```python
from build123d import *

# Parameters (mm, degrees)
SKETCH2_W                = 177.8
SKETCH2_H                = 165.1
BOSS_EXTRUDE1_DEPTH      = 25.4
SKETCH6_W                = 25.4
SKETCH6_H                = 25.4
BOSS_EXTRUDE2_DEPTH      = 31.75
MIRROR2_COPY_1_SKETCH_W  = 25.4
MIRROR2_COPY_1_SKETCH_H  = 25.4
MIRROR2_COPY_1_DEPTH     = 31.75
SKETCH9_W                = 107.188
SKETCH9_H                = 107.188
CUT_EXTRUDE3_DEPTH       = 3.556
SKETCH10_RX              = 2.159
SKETCH10_RY              = 2.159
CUT_EXTRUDE4_DEPTH       = 20.32
MIRROR4_COPY_1_SKETCH_RX = 2.159
MIRROR4_COPY_1_SKETCH_RY = 2.159
MIRROR4_COPY_1_DEPTH     = 20.32
SKETCH14_R               = 5.08
CUT_EXTRUDE5_DEPTH       = 20.32
MIRROR6_COPY_1_SKETCH_R  = 5.08
MIRROR6_COPY_1_DEPTH     = 20.32


with BuildPart() as part:
    # Sketch2 → Boss-Extrude1 (new body)
    with BuildSketch(Plane(origin=(0, 0, 0), x_dir=(1, 0, 0), z_dir=(0, 1, 0))):
        with Locations((88.9, -82.55)):
            Rectangle(SKETCH2_W, SKETCH2_H)
    extrude(amount=BOSS_EXTRUDE1_DEPTH)

    # Sketch6 → Boss-Extrude2 (add)
    with BuildSketch(Plane(origin=(0, 25.4, 0), x_dir=(1, 0, 0), z_dir=(0, 1, 0))):
        with Locations((12.7, -12.7)):
            Rectangle(SKETCH6_W, SKETCH6_H)
    boss_extrude2 = extrude(amount=BOSS_EXTRUDE2_DEPTH)

    # Mirror1: Boss-Extrude2 across plane
    add(boss_extrude2.mirror(Plane(origin=(0, 0, 82.55), x_dir=(1, 0, 0), z_dir=(0, 0, -1))))

    # Mirror2: Boss-Extrude2 across plane
    add(boss_extrude2.mirror(Plane.ZY.offset(-88.9)))

    # Mirror2 copy 1 sketch → Mirror2 copy 1 (add)
    with BuildSketch(Plane(origin=(177.8, 25.4, 165.1), x_dir=(-1, 0, 0), z_dir=(0, 1, 0))):
        with Locations((12.7, -12.7)):
            Rectangle(MIRROR2_COPY_1_SKETCH_W, MIRROR2_COPY_1_SKETCH_H)
    extrude(amount=MIRROR2_COPY_1_DEPTH)

    # Sketch9 → Cut-Extrude3 (cut)
    with BuildSketch(Plane(origin=(0, 25.4, 0), x_dir=(1, 0, 0), z_dir=(0, 1, 0))):
        with Locations((59.944, -81.276983136)):
            Rectangle(SKETCH9_W, SKETCH9_H)
    extrude(amount=-CUT_EXTRUDE3_DEPTH, mode=Mode.SUBTRACT)

    # Sketch10 → Cut-Extrude4 (cut)
    with BuildSketch(Plane(origin=(0, 21.844, 0), x_dir=(1, 0, 0), z_dir=(0, 1, 0))):
        with Locations(Location((9.662951288, -31.573935809), (0, 0, 56.28607255))):
            Ellipse(SKETCH10_RX, SKETCH10_RY)
    cut_extrude4 = extrude(amount=-CUT_EXTRUDE4_DEPTH, mode=Mode.SUBTRACT)

    # Mirror3: Cut-Extrude4 across plane
    add(cut_extrude4.mirror(Plane.XY.offset(81.276983136)), mode=Mode.SUBTRACT)

    # Mirror4: Cut-Extrude4 across plane
    add(cut_extrude4.mirror(Plane.ZY.offset(-59.944)), mode=Mode.SUBTRACT)

    # Mirror4 copy 1 sketch → Mirror4 copy 1 (cut)
    with BuildSketch(Plane(origin=(119.888, 21.844, 162.553966273), x_dir=(-1, 0, 0), z_dir=(0, 1, 0))):
        with Locations(Location((9.662951288, -31.573935809), (0, 0, 56.28607255))):
            Ellipse(MIRROR4_COPY_1_SKETCH_RX, MIRROR4_COPY_1_SKETCH_RY)
    extrude(amount=-MIRROR4_COPY_1_DEPTH, mode=Mode.SUBTRACT)

    # Sketch14 → Cut-Extrude5 (cut)
    with BuildSketch(Plane(origin=(0, 57.15, 0), x_dir=(1, 0, 0), z_dir=(0, 1, 0))):
        with Locations(Location((12.7, -12.7, 0), (0, 0, 270))):
            Circle(SKETCH14_R)
    cut_extrude5 = extrude(amount=-CUT_EXTRUDE5_DEPTH, mode=Mode.SUBTRACT)

    # Mirror5: Cut-Extrude5 across plane
    add(cut_extrude5.mirror(Plane.ZY.offset(-88.9)), mode=Mode.SUBTRACT)

    # Mirror6: Cut-Extrude5 across plane
    add(cut_extrude5.mirror(Plane(origin=(0, 0, 82.55), x_dir=(1, 0, 0), z_dir=(0, 0, -1))), mode=Mode.SUBTRACT)

    # Mirror6 copy 1 sketch → Mirror6 copy 1 (cut)
    with BuildSketch(Plane(origin=(177.8, 57.15, 165.1), x_dir=(-1, 0, 0), z_dir=(0, 1, 0))):
        with Locations(Location((12.7, -12.7, 0), (0, 0, 270))):
            Circle(MIRROR6_COPY_1_SKETCH_R)
    extrude(amount=-MIRROR6_COPY_1_DEPTH, mode=Mode.SUBTRACT)


solid = part.part
```
Could you check a few things on this model? Use its own coordinates, in mm. A direction names the side the tool comes from. Give positions to 0.01 mm unless a question says otherwise; leave off trailing zeros. Write each loop counter-clockwise with the first axis right and the second up, starting at its lowest first coordinate (ties: lowest second). Pieces come first, ordered by that corner, then holes. Notation, with made-up numbers: (67.5, 68) - (96.5, 68) arc R10 cw to (96.5, 78) - close; hole circle Ø8 at (43.25, 21). An arc over 180 degrees is marked (long way). One line per item, written item: value. Start each with the question number.
Item 1: Please list where these lines run through material, in increasing order: line 1 (X direction, y = 50.5, z = 152.4); line 2 (Z direction, x = 165, y = 46); line 3 (X direction, y = 49, z = 12). Write a range as from..to.
Item 2: Imagine slicing it at A-A, the plane y = 51. List the corners of the cut face in (x, z) for me, and give its area (3 significant figures).
Item 3: Which directions (+Z, -Z, +X, -X, +Y, -Y) give clear straight access to the entire face, cutting with the end or side of a thin tool? Please do faces 1 (the face through (13, 41, 25.4)), 2 (the face through (152.4, 41, 152)), 3 (the face through (59, 21.844, 81)).
Item 4: I'm going to push flat-ended pins straight in: pin 1 (5 mm diameter, centred on x = 10.5, z = 152, fed in from +Y); pin 2 (6 mm diameter, centred on x = 98.5, z = 91, fed in from +Y); pin 3 (2 mm diameter, centred on x = 10.5, z = 131, fed in from +Y). Where does each tip first touch, or does it pass through?
Item 5: Imagine slicing it at D-D, the plane x = 93. List the corners of the cut face in (y, z) for me.
Item 6: Imagine slicing it at B-B, the plane z = 105. List the corners of the cut face in (x, y) for me.
Item 7: Imagine slicing it at C-C, the plane y = 27.5. List the corners of the cut face in (x, z) for me.
Item 8: If we mould it in two halves opening along Z, with no side actions, what happens to faces 4 (the face through (90, 15, 0)), 5 (the face through (165, 36.83, 13)), 6 (the face through (152.4, 41, 13))? For each: +Z half, -Z half, draft (parallel to the pull), parting line (faces both ways), or undercut.
Geometry says:
1. line 1: 0..7.62, 17.78..25.4, 152.4..160.02, 170.18..177.8
1. line 2: 0..7.62, 17.78..25.4, 139.7..147.32, 157.48..165.1
1. line 3: 0..7.67, 17.73..25.4, 152.4..160.07, 170.13..177.8
2. outline: (0, 0) - (25.4, 0) - (25.4, 25.4) - (0, 25.4) - close; (0, 139.7) - (25.4, 139.7) - (25.4, 165.1) - (0, 165.1) - close; (152.4, 0) - (177.8, 0) - (177.8, 25.4) - (152.4, 25.4) - close; (152.4, 139.7) - (177.8, 139.7) - (177.8, 165.1) - (152.4, 165.1) - close; hole circle Ø10.16 at (12.7, 12.7); hole circle Ø10.16 at (12.7, 152.4); hole circle Ø10.16 at (165.1, 12.7); hole circle Ø10.16 at (165.1, 152.4)
2. area: 2,260 mm^2
3. face 1: +X, -X, +Y
3. face 2: +Z, -Z, +Y
3. face 3: +Y
4. pin 1: y = 36.83
4. pin 2: y = 21.84
4. pin 3: y = 1.52
5. outline: (0, 0) - (25.4, 0) - (25.4, 27.68) - (21.84, 27.68) - (21.84, 134.87) - (25.4, 134.87) - (25.4, 165.1) - (0, 165.1) - close
6. outline: (0, 0) - (177.8, 0) - (177.8, 25.4) - (113.54, 25.4) - (113.54, 21.84) - (6.35, 21.84) - (6.35, 25.4) - (0, 25.4) - close
7. outline: (0, 0) - (25.4, 0) - (25.4, 25.4) - (0, 25.4) - close; (0, 139.7) - (25.4, 139.7) - (25.4, 165.1) - (0, 165.1) - close; (152.4, 0) - (177.8, 0) - (177.8, 25.4) - (152.4, 25.4) - close; (152.4, 139.7) - (177.8, 139.7) - (177.8, 165.1) - (152.4, 165.1) - close
8. face 4: -Z half
8. face 5: undercut
8. face 6: draft
